Verification items for the finished model (mm, model axes). A direction names the side the tool comes from. Coordinates: 2 decimals unless noted, no trailing zeros. Order: outer loops, then holes, each group sorted by start corner. A loop starts at its lowest first (then second) coordinate and runs counter-clockwise, first axis right, second up. Notation, with made-up numbers: M 39.25,54.5 L 85.25,54.5 A17 cw 85.25,63.5 Z; hole C 65.25,23.5 d9. An arc over 180 degrees is marked long. Return JSON: item names as keys, results as strings.
```python
from build123d import *

# Parameters (mm, degrees)
SKICA1_R                 = 1.75
P_IDAT_VYSUNUT_M1_DEPTH  = 5
ZAOBLIT1_R               = 4
P_IDAT_VYSUNUT_M2_DEPTH  = 5
SKICA3_R                 = 1.05
ODEBRAT_VYSUNUT_M1_DEPTH = 6
ODEBRAT_VYSUNUT_M2_DEPTH = 6
ODEBRAT_VYSUNUT_M3_DEPTH = 6
SCALE1_SCALE             = 8


with BuildPart() as part:
    # Skica1 → Přidat vysunutím1 (new, symmetric)
    with BuildSketch(Plane.XY):
        with BuildLine():
            Line((0, 0), (0, 16))
            Line((0, 16), (23.5, 16))
            Line((23.5, 16), (23.5, 0))
            Line((23.5, 0), (28.5, 0))
            Line((28.5, 0), (74.768828107, 23.497329584))
            ThreePointArc((74.768828107, 23.497329584), (78.5, 22.196090729), (82.231171893, 23.497329584))
            Line((82.231171893, 23.497329584), (128.5, 0))
            Line((128.5, 0), (133.5, 0))
            Line((133.5, 0), (133.5, 16))
            Line((133.5, 16), (157, 16))
            Line((157, 16), (157, 0))
            Line((157, 0), (162, 0))
            Line((162, 0), (162, 21))
            Line((162, 21), (128.5, 21))
            Line((128.5, 21), (128.5, 5.607818541))
            Line((128.5, 5.607818541), (84.49517003, 27.955391095))
            ThreePointArc((84.49517003, 27.955391095), (78.5, 34.196090729), (72.50482997, 27.955391095))
            Line((72.50482997, 27.955391095), (28.5, 5.607818541))
            Line((28.5, 5.607818541), (28.5, 21))
            Line((28.5, 21), (-5, 21))
            Line((-5, 21), (-5, 0))
            Line((-5, 0), (0, 0))
        make_face()
        with Locations((78.5, 28.196090729)):
            Circle(SKICA1_R, mode=Mode.SUBTRACT)
    extrude(amount=P_IDAT_VYSUNUT_M1_DEPTH, both=True)

    # Zaoblit1
    zaoblit1_edges = [part.edges().sort_by_distance(p)[0] for p in [
        (-5, 21, 0),
        (162, 21, 0),
    ]]
    fillet(zaoblit1_edges, radius=ZAOBLIT1_R)

    # Skica2 → Přidat vysunutím2 (add, symmetric)
    with BuildSketch(Plane.XY):
        Polygon((28.5, 21), (65.117103916, 24.203581484), (60.341045967, 21.778090882), (28.5, 18.992360325), align=None)
    p_idat_vysunut_m2 = extrude(amount=P_IDAT_VYSUNUT_M2_DEPTH, both=True)

    # Zrcadlit1: Přidat vysunutím2 across plane
    add(p_idat_vysunut_m2.mirror(Plane.ZY.offset(-78.5)))

    # Skica3 → Odebrat vysunutím1 (cut)
    with BuildSketch(Plane.XZ):
        with Locations(Location((-1.75, 0, 0), (0, 0, 270))):
            Circle(SKICA3_R)
        with Locations(Location((25.25, 0, 0), (0, 0, 270))):
            Circle(SKICA3_R)
    odebrat_vysunut_m1 = extrude(amount=-ODEBRAT_VYSUNUT_M1_DEPTH, mode=Mode.SUBTRACT)

    # Zrcadlit2: Odebrat vysunutím1 across plane
    add(odebrat_vysunut_m1.mirror(Plane.ZY.offset(-78.5)), mode=Mode.SUBTRACT)

    # Skica4 → Odebrat vysunutím2 (cut)
    with BuildSketch(Plane.XY.offset(5)):
        Polygon((23.5, 16), (28.5, 16), (28.5, 13), (23.5, 8), align=None)
    odebrat_vysunut_m2 = extrude(amount=-ODEBRAT_VYSUNUT_M2_DEPTH, mode=Mode.SUBTRACT)

    # Zrcadlit3: Odebrat vysunutím2 across plane
    add(odebrat_vysunut_m2.mirror(Plane.ZY.offset(-78.5)), mode=Mode.SUBTRACT)

    # Skica5 → Odebrat vysunutím3 (cut)
    with BuildSketch(Plane.XY.offset(5)):
        Polygon((60.341045967, 21.778090882), (65.117103916, 24.203581484), (60.314461293, 23.783404699), (55.538403344, 21.357914097), align=None)
        Polygon((91.882896084, 24.203581484), (96.685538707, 23.783404699), (101.461596656, 21.357914097), (96.658954033, 21.778090882), align=None)
    extrude(amount=-ODEBRAT_VYSUNUT_M3_DEPTH, mode=Mode.SUBTRACT)


with BuildPart() as part_1:
    # Scale1: scaled about (78.5, 15.605763545, -0.066585977)
    add(part.part.scale(SCALE1_SCALE).moved(Location((-549.5, -109.240344815, 0.466101839))))


solid = part_1.part
```
Q1. Material ranges on line 1 along Y through (x, z) = (78.5, 16); line 2 along Z through (x, y) = (720.5, -81); line 3 along Y through (x, z) = (77.5, -31.5), recorded low to high.
Values:
{"line 1": "68.33 to 102.33, 130.33 to 164.33", "line 2": "-39.53 to -7.93, 8.87 to 40.47", "line 3": "68.34 to 102.36, 130.29 to 164.32"}
Q2. Go/stop test with flat-tipped pins: pin 1 (5 mm diameter, centred on y = 58.5, z = 18.5, fed in from +X); pin 2 (7 mm diameter, centred on x = -70.5, y = 68.5, fed in from +Z); pin 3 (1.5 mm diameter, centred on y = 116.5, z = 17, fed in from +X); pin 4 (18.5 mm diameter, centred on x = 724.5, z = -1, fed in from -Y). Record where each tip stops, or that it passes through.
Values:
{"pin 1": "x = 727.5", "pin 2": "z = -7.53", "pin 3": "x = 126.5", "pin 4": "y = -109.24"}
Q3. Cross-section at C-C, the plane x = 594. Record the boundary of the cut face in (y, z), and give its area (3 significant figures).
Values:
{"outline": "M 18.76,-39.53 L 58.76,-39.53 L 58.76,40.47 L 18.76,40.47 Z", "area": "3,200 mm^2"}
Q4. Tool access check on faces 4 (the face through (503, -6, -7.534)), 5 (the face through (478.5, -10, 1)), 6 (the face through (518.5, -60, -8)), 7 (the face through (-438, 58.76, 1)). Record the directions out of +Z, -Z, +X, -X, +Y, -Y that give a thin tool (end or side, any length) a straight path to the whole face; none if there is none.
Values:
{"face 4": "+Z", "face 5": "+Z, -Z", "face 6": "+Z, -Z, -Y", "face 7": "+Z, -Z, -X, +Y"}
Q5. Cross-section at A-A, the plane x = 78.5. Record the boundary of the cut face in (y, z).
Values:
{"outline": "M 68.33,-39.53 L 102.33,-39.53 L 102.33,40.47 L 68.33,40.47 Z; M 130.33,-39.53 L 164.33,-39.53 L 164.33,40.47 L 130.33,40.47 Z"}
Q6. Cross-section at B-B, the plane z = -26.5. State how many separate pieces and enclosed holes the cut face has, and give its area (3 significant figures).
Values:
{"separate pieces": "1", "enclosed holes": "3", "area": "89,100 mm^2"}
Q7. Draft check along X on faces 1 (the face through (-139.02, -16.57, 1.03)), 2 (the face through (-580.37, 49.14, -0.09)), 3 (the face through (581, 22, 40.466)). Enter one of: pulls with the +X half, pulls with the -X half, needs draft (parallel to the pull), parting line crosses it, or undercut.
Values:
{"face 1": "undercut", "face 2": "pulls with the -X half", "face 3": "needs draft"}
